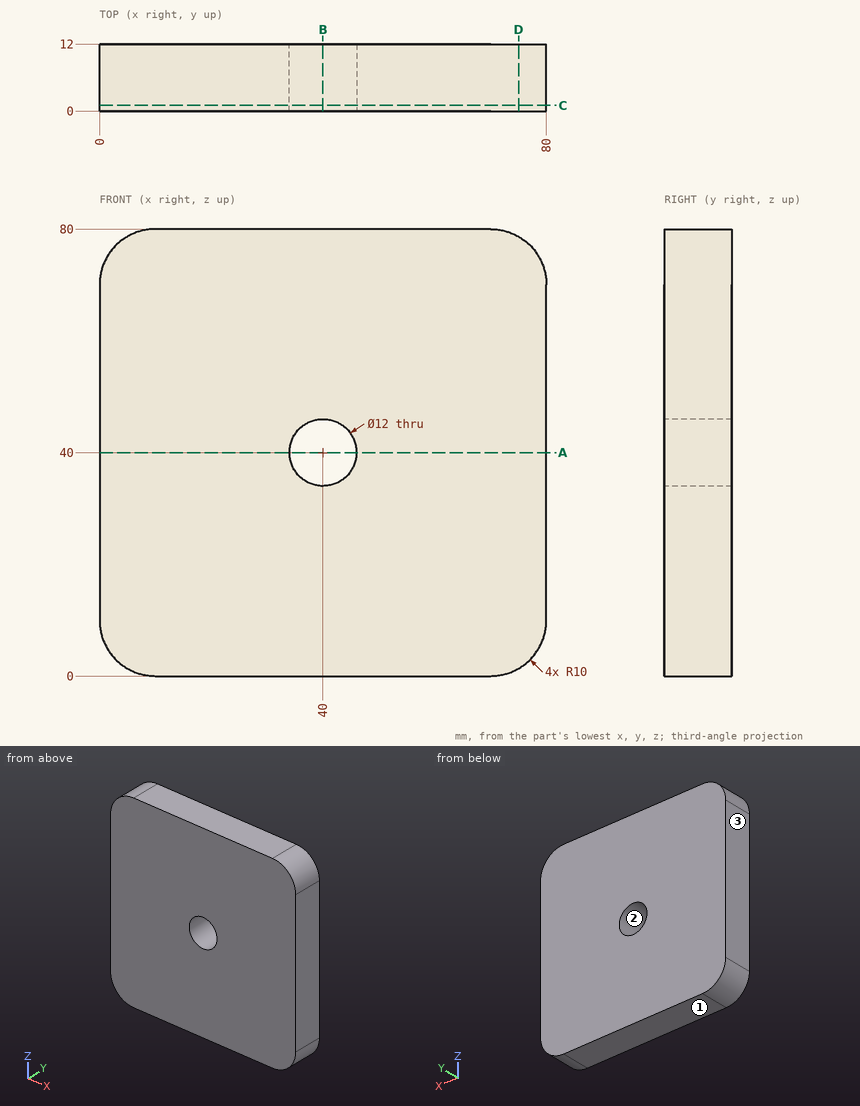
Job drawing, mm, ordinate dimensions from the low corner. One solid piece. Coordinates: 2 decimals unless noted, no trailing zeros. Write each loop counter-clockwise with the first axis right and the second up, starting at its lowest first coordinate (ties: lowest second). Pieces come first, ordered by that corner, then holes.
Item 1: Slice it at A-A (z = 40). Write the cut outline in (x, y).
Item 2: Slice it at C-C (y = 1). Write the cut outline in (x, z).
Item 3: Probe line 1 (Z direction, x = 40, y = 3.75); line 2 (X direction, y = 7, z = 41); line 3 (X direction, y = 1.25, z = 36.5). List the from-to ranges inside material, lowest first.
Item 4: Mould opens along Z. For the marked faces 1, 2 and 3 say: released by +Z, released by -Z, zero draft, split by the parting line, or undercut.
Item 5: Slice it at B-B (x = 40). Write the cut outline in (y, z), and give its area (3 significant figures).
Item 6: Slice it at D-D (x = 75). Write the cut outline in (y, z).
Results found:
1. outline: (0, 0) - (34, 0) - (34, 12) - (0, 12) - close; (46, 0) - (80, 0) - (80, 12) - (46, 12) - close
2. outline: (0, 10) arc R10 ccw to (10, 0) - (70, 0) arc R10 ccw to (80, 10) - (80, 70) arc R10 ccw to (70, 80) - (10, 80) arc R10 ccw to (0, 70) - close; hole circle Ø12 at (40, 40)
3. line 1: z = 0 to 34, 46 to 80
3. line 2: x = 0 to 34.08, 45.92 to 80
3. line 3: x = 0 to 35.13, 44.87 to 80
4. face 1: released by -Z
4. face 2: undercut
4. face 3: zero draft
5. outline: (0, 0) - (12, 0) - (12, 34) - (0, 34) - close; (0, 46) - (12, 46) - (12, 80) - (0, 80) - close
5. area: 816 mm2
6. outline: (0, 1.34) - (12, 1.34) - (12, 78.66) - (0, 78.66) - close
